The listing builds one solid part. Answer for the finished solid, in the listing's coordinates (mm). A direction names the side the tool comes from. Round coordinates to 2 decimals unless told otherwise and drop trailing zeros. Loops run counter-clockwise (first coordinate to the right, second up) from the corner with the lowest first, then second, coordinate; pieces in that order, holes last. Notation, with made-up numbers: (3, 55) - (10, 55) arc R24 ccw to (10, 66) - close; hole circle Ø1 at (-27.5, -3.75). An arc over 180 degrees is marked (long way). One line per item, written item: value.
Autodesk Inventor part; units mm, degrees
ref_plane "YZ Plane" through (0, 0, 0) normal (1, 0, 0) x (0, 1, 0)
ref_plane "XZ Plane" through (0, 0, 0) normal (0, 1, 0) x (-1, 0, 0)
ref_plane "XY Plane" through (0, 0, 0) normal (0, 0, 1) x (1, 0, 0)
sketch "Sketch1" plane through (0, 0, 0) normal (0, 0, 1) x (1, 0, 0)
  line L0 (0, 0) -> (165.1, 0)
  line L1 (165.1, 0) -> (165.1, 101.6)
  line L2 (165.1, 101.6) -> (0, 101.6)
  line L3 (0, 101.6) -> (0, 0)
  line L4 (0, 0) -> (57.15, 0)
  line L5 (57.15, 0) -> (57.15, 12.7)
  line L6 (57.15, 12.7) -> (0, 12.7)
  line L7 (0, 12.7) -> (0, 0)
  line L8 (165.1, 0) -> (107.95, 0)
  line L9 (107.95, 0) -> (107.95, 12.7)
  line L10 (107.95, 12.7) -> (165.1, 12.7)
  line L11 (165.1, 12.7) -> (165.1, 0)
  line L12 (0, 12.7) -> (12.7, 12.7)
  line L13 (12.7, 12.7) -> (12.7, 34.925)
  line L14 (12.7, 34.925) -> (0, 34.925)
  line L15 (0, 34.925) -> (0, 12.7)
  line L16 (165.1, 12.7) -> (152.4, 12.7)
  line L17 (152.4, 12.7) -> (152.4, 34.925)
  line L18 (152.4, 34.925) -> (165.1, 34.925)
  line L19 (165.1, 34.925) -> (165.1, 12.7)
  line L20 (0, 101.6) -> (12.7, 101.6)
  line L21 (12.7, 101.6) -> (12.7, 66.675)
  line L22 (12.7, 66.675) -> (0, 66.675)
  line L23 (0, 66.675) -> (0, 101.6)
  line L24 (165.1, 101.6) -> (152.4, 101.6)
  line L25 (152.4, 101.6) -> (152.4, 66.675)
  line L26 (152.4, 66.675) -> (165.1, 66.675)
  line L27 (165.1, 66.675) -> (165.1, 101.6)
  point P0 (0, 66.675)
  point P1 (0, 34.925)
  dimension "d0" = 101.6
  dimension "d1" = 165.1
  dimension "d2" = 57.15
  dimension "d3" = 12.7
  dimension "d4" = 57.15
  dimension "d5" = 12.7
  dimension "d6" = 12.7
  dimension "d7" = 22.225
  dimension "d8" = 12.7
  dimension "d9" = 22.225
  dimension "d10" = 12.7
  dimension "d11" = 34.925
  dimension "d12" = 12.7
  dimension "d13" = 34.925
extrude "Extrusion1" add sketch "Sketch1" along normal blind 12.7 contours L5 L6 L13 L14 L3 L22 L21 L2 L25 L26 L1 L18 L17 L10 L9 L0
sketch "Sketch2" plane through (0, 0, 12.7) normal (0, 0, 1) x (1, 0, 0)
  line L0 (12.7, 66.675) -> (0, 66.675)
  line L1 (12.7, 66.675) -> (10.4549, 68.9201)
  line L2 (12.7, 101.6) -> (12.7, 66.675)
  line L3 (12.7, 34.925) -> (12.7, 12.7)
  line L4 (12.7, 34.925) -> (10.4549, 32.6799)
  line L5 (57.15, 12.7) -> (57.15, 0)
  line L6 (57.15, 12.7) -> (54.9049, 10.4549)
  line L7 (107.95, 0) -> (107.95, 12.7)
  line L8 (107.95, 12.7) -> (110.1951, 10.4549)
  line L9 (107.95, 12.7) -> (152.4, 12.7)
  line L10 (152.4, 12.7) -> (152.4, 34.925)
  line L11 (152.4, 34.925) -> (154.6451, 32.6799)
  line L12 (152.4, 34.925) -> (165.1, 34.925)
  line L13 (165.1, 66.675) -> (152.4, 66.675)
  line L14 (152.4, 66.675) -> (154.6451, 68.9201)
  circle A0 centre (10.4549, 68.9201) radius 3.175
  circle A1 centre (10.4549, 32.6799) radius 3.175
  circle A2 centre (54.9049, 10.4549) radius 3.175
  circle A3 centre (110.1951, 10.4549) radius 3.175
  circle A4 centre (154.6451, 32.6799) radius 3.175
  circle A5 centre (154.6451, 68.9201) radius 3.175
  point P0 (0, 0)
  dimension "d16" = 3.175
  dimension "d17" = 45
  dimension "d18" = 3.175
  dimension "d19" = 45
  dimension "d20" = 3.175
  dimension "d21" = 45
  dimension "d22" = 3.175
  dimension "d23" = 45
  dimension "d24" = 3.175
  dimension "d25" = 45
  dimension "d26" = 3.175
  dimension "d27" = 45
  dimension "d28" = 6.35
  dimension "d29" = 6.35
  dimension "d30" = 6.35
  dimension "d31" = 6.35
  dimension "d32" = 6.35
  dimension "d33" = 6.35
extrude "Extrusion2" cut sketch "Sketch2" against normal blind 12.7
sketch "Sketch4" plane through (0, 0, 12.7) normal (0, 0, 1) x (1, 0, 0)
  circle A0 centre (22.225, 82.55) radius 3.175
  circle A1 centre (22.225, 57.15) radius 3.175
  line L0 (12.7, 101.6) -> (12.7, 71.1651)
  circle A2 centre (22.225, 31.75) radius 3.175
  line L1 (12.7, 30.4349) -> (12.7, 12.7)
  line L2 (57.15, 0) -> (107.95, 0)
  circle A3 centre (142.875, 31.75) radius 3.175
  circle A4 centre (142.875, 57.15) radius 3.175
  circle A5 centre (142.875, 82.55) radius 3.175
  line L3 (152.4, 71.1651) -> (152.4, 101.6)
  line L4 (152.4, 12.7) -> (152.4, 30.4349)
  circle A6 centre (82.55, 22.225) radius 3.175
  line L5 (112.4401, 12.7) -> (152.4, 12.7)
  line L6 (57.15, 8.2099) -> (57.15, 0)
  circle A7 centre (57.15, 22.225) radius 3.175
  line L7 (12.7, 12.7) -> (52.6599, 12.7)
  circle A8 centre (107.95, 22.225) radius 3.175
  point P0 (0, 0)
  dimension "d63" = 6.35
  dimension "d64" = 6.35
  dimension "d65" = 9.525
  dimension "d66" = 9.525
  dimension "d67" = 6.35
  dimension "d68" = 9.525
  dimension "d69" = 31.75
  dimension "d70" = 25.4
  dimension "d71" = 25.4
  dimension "d72" = 6.35
  dimension "d73" = 6.35
  dimension "d74" = 6.35
  dimension "d75" = 9.525
  dimension "d76" = 9.525
  dimension "d77" = 9.525
  dimension "d78" = 31.75
  dimension "d79" = 25.4
  dimension "d80" = 25.4
  dimension "d81" = 6.35
  dimension "d82" = 9.525
  dimension "d83" = 25.4
  dimension "d84" = 6.35
  dimension "d85" = 9.525
  dimension "d86" = 25.4
  dimension "d87" = 6.35
  dimension "d88" = 25.4
  dimension "d89" = 9.525
extrude "Extrusion4" cut sketch "Sketch4" against normal blind 12.7
sketch "Sketch5" plane through (0, 0, 12.7) normal (0, 0, 1) x (1, 0, 0)
  circle A0 centre (22.225, 76.2) radius 3.175
  circle A1 centre (22.225, 82.55) radius 3.175
  circle A2 centre (22.225, 50.8) radius 3.175
  circle A3 centre (22.225, 25.4) radius 3.175
  line L0 (12.7, 101.6) -> (12.7, 71.1651)
  point P0 (0, 0)
  dimension "d92" = 6.35
  dimension "d93" = 6.35
  dimension "d94" = 6.35
  dimension "d95" = 6.35
  dimension "d96" = 9.525
  dimension "d97" = 9.525
  dimension "d98" = 9.525
  dimension "d99" = 25.4
  dimension "d100" = 25.4
extrude "Extrusion5" cut sketch "Sketch5" against normal blind 12.7 contours A0 | A2 | A3
sketch "Sketch6" plane through (0, 0, 12.7) normal (0, 0, 1) x (1, 0, 0)
  circle A0 centre (22.225, 82.55) radius 3.175
  circle A1 centre (22.225, 82.55) radius 3.175
  circle A2 centre (22.225, 57.15) radius 3.175
  circle A3 centre (22.225, 57.15) radius 3.175
  circle A4 centre (22.225, 31.75) radius 3.175
  circle A5 centre (22.225, 31.75) radius 3.175
  point P0 (0, 0)
  point P1 (22.225, 79.375)
  point P2 (22.225, 53.975)
  point P3 (22.225, 28.575)
  dimension "d103" = 6.35
  dimension "d104" = 6.35
  dimension "d105" = 6.35
extrude "Extrusion6" add sketch "Sketch6" against normal blind 12.7
sketch "Sketch8" plane through (0, 0, 12.7) normal (0, 0, 1) x (1, 0, 0)
  circle A0 centre (142.875, 82.55) radius 3.175
  circle A1 centre (142.875, 82.55) radius 3.175
  circle A2 centre (142.875, 57.15) radius 3.175
  circle A3 centre (142.875, 57.15) radius 3.175
  circle A4 centre (142.875, 31.75) radius 3.175
  circle A5 centre (142.875, 31.75) radius 3.175
  point P0 (0, 0)
  dimension "d116" = 6.35
  dimension "d117" = 6.35
  dimension "d118" = 6.35
extrude "Extrusion8" add sketch "Sketch8" against normal blind 12.7
sketch "Sketch11" plane through (0, 0, 12.7) normal (0, 0, 1) x (1, 0, 0)
  circle A0 centre (69.85, 22.225) radius 3.175
  circle A1 centre (95.25, 22.225) radius 3.175
  line L0 (12.7, 12.7) -> (52.6599, 12.7)
  line L1 (112.4401, 12.7) -> (152.4, 12.7)
  line L2 (57.15, 8.2099) -> (57.15, 0)
  line L3 (107.95, 0) -> (107.95, 8.2099)
  point P0 (0, 0)
  dimension "d132" = 6.35
  dimension "d133" = 6.35
  dimension "d134" = 9.525
  dimension "d135" = 9.525
  dimension "d136" = 12.7
  dimension "d137" = 12.7
extrude "Extrusion10" cut sketch "Sketch11" against normal blind 12.7
sketch "Sketch12" plane through (0, 0, 12.7) normal (0, 0, 1) x (1, 0, 0)
  circle A0 centre (82.55, 22.225) radius 3.175
  circle A1 centre (82.55, 22.225) radius 3.175
  circle A2 centre (57.15, 22.225) radius 3.175
  circle A3 centre (57.15, 22.225) radius 3.175
  circle A4 centre (107.95, 22.225) radius 3.175
  circle A5 centre (107.95, 22.225) radius 3.175
  point P0 (0, 0)
  dimension "d140" = 6.35
  dimension "d141" = 6.35
  dimension "d142" = 6.35
extrude "Extrusion11" add sketch "Sketch12" against normal blind 12.7
sketch "Sketch13" plane through (0, 0, 12.7) normal (0, 0, 1) x (1, 0, 0)
  circle A0 centre (69.85, 92.075) radius 3.175
  circle A1 centre (95.25, 92.075) radius 3.175
  line L0 (152.4, 101.6) -> (12.7, 101.6)
  line L1 (57.15, 8.2099) -> (57.15, 0)
  point P0 (0, 0)
  dimension "d145" = 6.35
  dimension "d146" = 6.35
  dimension "d147" = 9.525
  dimension "d148" = 9.525
  dimension "d149" = 25.4
  dimension "d150" = 12.7
extrude "Extrusion12" cut sketch "Sketch13" against normal blind 12.7
sketch "Sketch14" plane through (0, 0, 12.7) normal (0, 0, 1) x (1, 0, 0)
  line L0 (57.15, 0) -> (107.95, 0)
  line L1 (152.4, 12.7) -> (152.4, 30.4349)
  circle A0 centre (142.875, 38.1) radius 3.175
  circle A1 centre (142.875, 63.5) radius 3.175
  point P0 (0, 0)
  dimension "d156" = 6.35
  dimension "d158" = 6.35
  dimension "d160" = 9.525
  dimension "d161" = 9.525
  dimension "d162" = 25.4
  dimension "d165" = 38.1
extrude "Extrusion13" cut sketch "Sketch14" against normal blind 12.7
properties part number "Front Wall"
1) For faces 1 (the flat face through (33, 12.7, 6)), 2 (the cylindrical face through (152.45, 34.974, 6.439)), 3 (the flat face through (152.4, 21, 6)), 4 (the flat face through (152.4, 87, 6)), 5 (the flat face through (12.7, 87, 6)), determine the directions among +Z, -Z, +X, -X, +Y, -Y from which every point of the face is accessible in a straight line to the end or side of a thin tool.
Final values:
face 1: +Z, -Z, -X, -Y
face 2: +Z, -Z
face 3: +Z, -Z, +X, -Y
face 4: +Z, -Z, +X, +Y
face 5: +Z, -Z, -X, +Y
2) A cutting plane is placed at D-D on x = 121.5. Give the vertices of the cut face in (y, z).
Final values:
outline: (12.7, 0) - (101.6, 0) - (101.6, 12.7) - (12.7, 12.7) - close
3) For a pull along Y with two mould halves and no side action, classify faces 6 (the flat face through (82, 0, 6)), 7 (the flat face through (161, 66.675, 6)), 8 (the cylindrical face through (140.535, 65.646, 6.439)), 9 (the cylindrical face through (12.749, 34.875, 6.439)) as released by +Y, released by -Y, zero draft, split by the parting line, or undercut.
Final values:
face 6: released by -Y
face 7: released by +Y
face 8: undercut
face 9: undercut
4) Consider L1, parallel to X at y = 22, z = 4; L2, parallel to Y at x = 95.25, z = 9.75; L3, parallel to X at y = 23.5, z = 6. Determine where each line is inside the solid, lowest interval first.
Final values:
L1: 12.7 to 66.68, 73.02 to 92.08, 98.42 to 152.4
L2: 0 to 19.05, 25.4 to 88.9, 95.25 to 101.6
L3: 12.7 to 19.68, 24.77 to 66.94, 72.76 to 92.34, 98.16 to 152.4
5) A cutting plane is placed at A-A on x = 69.85. Give the vertices of the cut face in (y, z).
Final values:
outline: (0, 0) - (19.05, 0) - (19.05, 12.7) - (0, 12.7) - close; (25.4, 0) - (88.9, 0) - (88.9, 12.7) - (25.4, 12.7) - close; (95.25, 0) - (101.6, 0) - (101.6, 12.7) - (95.25, 12.7) - close
6) Each of these flat-tipped pins is pushed along its axis until it touches: pin 1 Ø4 at (x, y) = (142.875, 63.5) entering from -Z; pin 2 Ø4 at (y, z) = (26, 10.5) entering from +X; pin 3 Ø7.5 at (x, y) = (95.25, 92.075) entering from -Z; pin 4 Ø6.5 at (y, z) = (84, 8) entering from -X. Where does it stop, or does it pass through?
Final values:
pin 1: through
pin 2: x = 152.4
pin 3: z = 0
pin 4: x = 12.7
7) A cutting plane is placed at C-C on z = 10.5. Give the number of separate pieces and of enclosed holes in the cut face, and give its area (3 significant figures).
Final values:
separate pieces: 1
enclosed holes: 9
area: 13,600 mm2
8) A cutting plane is placed at B-B on y = 38.1. Give the vertices of the cut face in (x, z).
Final values:
outline: (0, 0) - (139.7, 0) - (139.7, 12.7) - (0, 12.7) - close; (146.05, 0) - (165.1, 0) - (165.1, 12.7) - (146.05, 12.7) - close
